For this review, take the finished solid that the model builds, in its own axes (mm). A direction names the side the tool comes from. Round coordinates to 2 decimals unless told otherwise and drop trailing zeros. Write each question's results on one line, items separated by ' | '. Start each with the question number.
Item 1: Add section A-A (y = 0.75). Count the separate pieces of the cut face and the enclosed holes in it, plus the area to 3 significant figures.
Item 2: The part is to be moulded in two halves that separate along Z. For faces 1 (the cylindrical face through (17.662, 0.74, 6.257)), 2 (the flat face through (-12.761, 1, -15)), 3 (the cylindrical face through (-20.9, 0.74, 18.43)), say which applies: +Z half, -Z half, draft (parallel to the pull), parting line (faces both ways), or undercut.
Item 3: To check wall thickness, follow line 1 along Z through (x, y) = (8.5, 0.35); line 2 along Z through (x, y) = (-20, 1.25); line 3 along X through (y, z) = (1.15, -6.5). State the ranges of each line that lie inside material, in increasing order.
Item 4: Tool access review of faces 4 (the flat face through (-1.365, 1, -15)), 5 (the flat face through (0, 1.5, 0)): name each direction out of +Z, -Z, +X, -X, +Y, -Y from which nothing blocks a thin tool from reaching the whole face with its end or side.
Item 5: Clearance check with flat-ended pins moving along their axes: pin 1 (0.9 mm diameter, centred on x = 0.91, z = 15.19, fed in from +Y); pin 2 (0.8 mm diameter, centred on y = 0.5, z = -18.5, fed in from +X). State where each tip first meets the part, or that it passes through.
from build123d import *

# Parameters (mm, degrees)
BOSS_EXTRUDE1_DEPTH = 1.5
CAVITY1_START       = -19
CAVITY1_DEPTH       = 6.2
CAVITY1_2_DEPTH     = 2.01
CUT_EXTRUDE3_REACH  = 30.732
SKETCH5_R           = 1.1
CUT_EXTRUDE6_DEPTH  = 1.5
SKETCH6_W           = 2.5
SKETCH6_H           = 6.3
CUT_EXTRUDE7_DEPTH  = 0.01
SKETCH7_R           = 0.75
CUT_EXTRUDE8_DEPTH  = 1.5
SKETCH8_OUTSIDE_W   = 56.48
SKETCH8_OUTSIDE_H   = 51.48
SKETCH8_OUTSIDE_R   = 0.555
CUT_EXTRUDE9_DEPTH  = 1.5
SKETCH9_R           = 0.75
SKETCH9_R_2         = 0.508
SKETCH9_R_3         = 0.262351118
CUT_EXTRUDE10_DEPTH = 1.5


# Read off the part's stored shape, not the designer's step: Cavity1
with BuildPart() as part:
    # Sketch1 → Boss-Extrude1 (new body)
    with BuildSketch(Plane(origin=(0, 0, 0), x_dir=(1, 0, 0), z_dir=(0, 1, 0))):
        with BuildLine():
            Line((-19.5, 19), (19.5, 19))
            ThreePointArc((19.5, 19), (20.914213562, 18.414213562), (21.5, 17))
            Line((21.5, 17), (21.5, -17))
            ThreePointArc((21.5, -17), (20.914213562, -18.414213562), (19.5, -19))
            Line((19.5, -19), (-19.5, -19))
            ThreePointArc((-19.5, -19), (-20.914213562, -18.414213562), (-21.5, -17))
            Line((-21.5, -17), (-21.5, 17))
            ThreePointArc((-21.5, 17), (-20.914213562, 18.414213562), (-19.5, 19))
        make_face()
    extrude(amount=BOSS_EXTRUDE1_DEPTH)

    # Cavity1 outline → Cavity1 (cut)
    with BuildSketch(Plane.XY.offset(CAVITY1_START)):
        with BuildLine():
            ThreePointArc((-11.428721681, 1.5), (-12.051521733, 0.792798554), (-12.560917691, 0))
            Line((-12.560917691, 0), (-1.565146914, 0))
            ThreePointArc((-1.565146914, 0), (-2.074542872, 0.792798554), (-2.697342924, 1.5))
            Line((-2.697342924, 1.5), (-11.428721681, 1.5))
        make_face()
    extrude(amount=CAVITY1_DEPTH, mode=Mode.SUBTRACT)

    # Cavity1 2 outline → Cavity1 2 (cut)
    with BuildSketch(Plane.XY.offset(CAVITY1_START)):
        with BuildLine():
            Line((-17.158032303, 1.5), (-17.158032303, 0))
            Line((-17.158032303, 0), (-12.560917691, 0))
            ThreePointArc((-12.560917691, 0), (-12.051521733, 0.792798554), (-11.428721681, 1.5))
            Line((-11.428721681, 1.5), (-17.158032303, 1.5))
        make_face()
        with BuildLine():
            ThreePointArc((-2.697342924, 1.5), (-2.074542872, 0.792798554), (-1.565146914, 0))
            Line((-1.565146914, 0), (3.031967697, 0))
            Line((3.031967697, 0), (3.031967697, 1.5))
            Line((3.031967697, 1.5), (-2.697342924, 1.5))
        make_face()
    extrude(amount=CAVITY1_2_DEPTH, mode=Mode.SUBTRACT)

    # Cut-Extrude3: up to this face of the body (flat: up to its plane)
    cut_extrude3_end = Plane(part.part.faces().sort_by_distance((0.396422331, 0, 0.917486048))[0])
    # Sketch4 → Cut-Extrude3 (cut, up to the picked face)
    with BuildSketch(Plane(origin=(0, 1.5, 0), x_dir=(1, 0, 0), z_dir=(0, 1, 0)), mode=Mode.PRIVATE) as cut_extrude3_sk1:
        with BuildLine():
            Line((-16.858032303, 16.79), (-13.060917691, 16.79))
            ThreePointArc((-13.060917691, 16.79), (-12.848785657, 16.702132034), (-12.760917691, 16.49))
            Line((-12.760917691, 16.49), (-12.760917691, 13.3))
            ThreePointArc((-12.760917691, 13.3), (-12.555892438, 12.805025253), (-12.060917691, 12.6))
            Line((-12.060917691, 12.6), (-2.065146914, 12.6))
            ThreePointArc((-2.065146914, 12.6), (-1.570172167, 12.805025253), (-1.365146914, 13.3))
            Line((-1.365146914, 13.3), (-1.365146914, 16.49))
            ThreePointArc((-1.365146914, 16.49), (-1.277278948, 16.702132034), (-1.065146914, 16.79))
            Line((-1.065146914, 16.79), (2.739051684, 16.79))
            ThreePointArc((2.739051684, 16.79), (3.08759594, 16.934371758), (3.231967697, 17.282916013))
            Line((3.231967697, 17.282916013), (3.231967697, 19.2))
            Line((3.231967697, 19.2), (-17.358032303, 19.2))
            Line((-17.358032303, 19.2), (-17.358032303, 17.29))
            ThreePointArc((-17.358032303, 17.29), (-17.211585693, 16.936446609), (-16.858032303, 16.79))
        make_face()
    cut_extrude3_tool1 = split(extrude(cut_extrude3_sk1.sketch, amount=-CUT_EXTRUDE3_REACH, mode=Mode.PRIVATE), bisect_by=cut_extrude3_end, keep=Keep.BOTH, mode=Mode.PRIVATE)
    add(cut_extrude3_tool1.solids().sort_by(Axis((-7.062875, 1.5, -16.384158), (0, -1, 0)))[0], mode=Mode.SUBTRACT)

    # Sketch5 → Cut-Extrude6 (cut)
    with BuildSketch(Plane(origin=(0, 1.5, 0), x_dir=(1, 0, 0), z_dir=(0, 1, 0))):
        with Locations(Location((19.5, 17, 0), (0, 0, 270))):
            Circle(SKETCH5_R)
        with Locations(Location((19.5, -17, 0), (0, 0, 270))):
            Circle(SKETCH5_R)
        with Locations(Location((-19.5, 17, 0), (0, 0, 270))):
            Circle(SKETCH5_R)
        with Locations(Location((-19.5, -17, 0), (0, 0, 270))):
            Circle(SKETCH5_R)
    extrude(amount=-CUT_EXTRUDE6_DEPTH, mode=Mode.SUBTRACT)

    # Sketch6 → Cut-Extrude7 (cut)
    with BuildSketch(Plane.XZ):
        with Locations((-10.046489819, -9.45)):
            Rectangle(SKETCH6_W, SKETCH6_H)
        with Locations((-4.079574786, -9.45)):
            Rectangle(SKETCH6_W, SKETCH6_H)
    extrude(amount=-CUT_EXTRUDE7_DEPTH, mode=Mode.SUBTRACT)

    # Sketch7 → Cut-Extrude8 (cut)
    with BuildSketch(Plane(origin=(0, 1.5, 0), x_dir=(1, 0, 0), z_dir=(0, 1, 0))):
        with Locations(Location((-13, 8.22889094, 0), (0, 0, 270))):
            Circle(SKETCH7_R)
        with Locations(Location((-19, 8.22889094, 0), (0, 0, 270))):
            Circle(SKETCH7_R)
    extrude(amount=-CUT_EXTRUDE8_DEPTH, mode=Mode.SUBTRACT)

    # Sketch8 outside → Cut-Extrude9 (cut)
    # profile 1 of 3: a face of its own
    with BuildSketch(Plane(origin=(0, 1.5, 0), x_dir=(1, 0, 0), z_dir=(0, 1, 0))):
        Rectangle(SKETCH8_OUTSIDE_W, SKETCH8_OUTSIDE_H)
        with BuildLine():
            Line((-17.358032303, 17.29), (-17.358032303, 19))
            Line((-17.358032303, 19), (-19.5, 19))
            ThreePointArc((-19.5, 19), (-20.914213562, 18.414213562), (-21.5, 17))
            Line((-21.5, 17), (-21.5, -17))
            ThreePointArc((-21.5, -17), (-20.914213562, -18.414213562), (-19.5, -19))
            Line((-19.5, -19), (19.5, -19))
            ThreePointArc((19.5, -19), (20.914213562, -18.414213562), (21.5, -17))
            Line((21.5, -17), (21.5, 17))
            ThreePointArc((21.5, 17), (20.914213562, 18.414213562), (19.5, 19))
            Line((19.5, 19), (3.231967697, 19))
            Line((3.231967697, 19), (3.231967697, 17.282916013))
            ThreePointArc((3.231967697, 17.282916013), (3.08759594, 16.934371758), (2.739051684, 16.79))
            Line((2.739051684, 16.79), (-1.065146914, 16.79))
            ThreePointArc((-1.065146914, 16.79), (-1.277278948, 16.702132034), (-1.365146914, 16.49))
            Line((-1.365146914, 16.49), (-1.365146914, 13.3))
            ThreePointArc((-1.365146914, 13.3), (-1.570172167, 12.805025253), (-2.065146914, 12.6))
            Line((-2.065146914, 12.6), (-12.060917691, 12.6))
            ThreePointArc((-12.060917691, 12.6), (-12.555892438, 12.805025253), (-12.760917691, 13.3))
            Line((-12.760917691, 13.3), (-12.760917691, 16.49))
            ThreePointArc((-12.760917691, 16.49), (-12.848785657, 16.702132034), (-13.060917691, 16.79))
            Line((-13.060917691, 16.79), (-16.858032303, 16.79))
            ThreePointArc((-16.858032303, 16.79), (-17.211585693, 16.936446609), (-17.358032303, 17.29))
        make_face(mode=Mode.SUBTRACT)
    # profile 2 of 3: a face of its own
    with BuildSketch(Plane(origin=(0, 1.5, 0), x_dir=(1, 0, 0), z_dir=(0, 1, 0))):
        with Locations(Location((-12.744728974, -16.255, 0), (0, 0, 270))):
            Circle(SKETCH8_OUTSIDE_R)
    # profile 3 of 3: a face of its own
    with BuildSketch(Plane(origin=(0, 1.5, 0), x_dir=(1, 0, 0), z_dir=(0, 1, 0))):
        with Locations(Location((-9.284728974, -16.255, 0), (0, 0, 270))):
            Circle(SKETCH8_OUTSIDE_R)
    extrude(amount=-CUT_EXTRUDE9_DEPTH, mode=Mode.SUBTRACT)

    # Sketch9 → Cut-Extrude10 (cut)
    with BuildSketch(Plane.XZ):
        with Locations(Location((8.53007963, -8.501636461, 0), (0, 0, 270))):
            Circle(SKETCH9_R)
        with Locations(Location((18.158240781, 11.226709095, 0), (0, 0, 270))):
            Circle(SKETCH9_R_2)
        with Locations(Location((18.158240781, 8.686709095, 0), (0, 0, 270))):
            Circle(SKETCH9_R_2)
        with Locations(Location((18.158240781, 6.146709095, 0), (0, 0, 270))):
            Circle(SKETCH9_R_2)
        with Locations(Location((18.158240781, 3.606709095, 0), (0, 0, 270))):
            Circle(SKETCH9_R_2)
        with Locations(Location((16.15007963, 15.19, 0), (0, 0, 270))):
            Circle(SKETCH9_R_2)
        with Locations(Location((-7.063032303, -6.3, 0), (0, 0, 270))):
            Circle(SKETCH9_R_3)
        with Locations(Location((0.91007963, 15.19, 0), (0, 0, 270))):
            Circle(SKETCH9_R_2)
    extrude(amount=-CUT_EXTRUDE10_DEPTH, mode=Mode.SUBTRACT)


solid = part.part
Responses:
1) separate pieces: 1 | enclosed holes: 16 | area: 1,510 mm^2
2) face 1: undercut | face 2: draft | face 3: +Z half
3) line 1: z = -19 to -9.25, -7.75 to 19 | line 2: z = -18.94 to -17.98, -16.02 to 16.02, 17.98 to 18.94 | line 3: x = -21.5 to -7.23, -6.89 to 21.5
4) face 4: -Z, +Y, -Y | face 5: +Z, -Z, +X, -X, +Y
5) pin 1: passes through | pin 2: stops at x = 21.17
